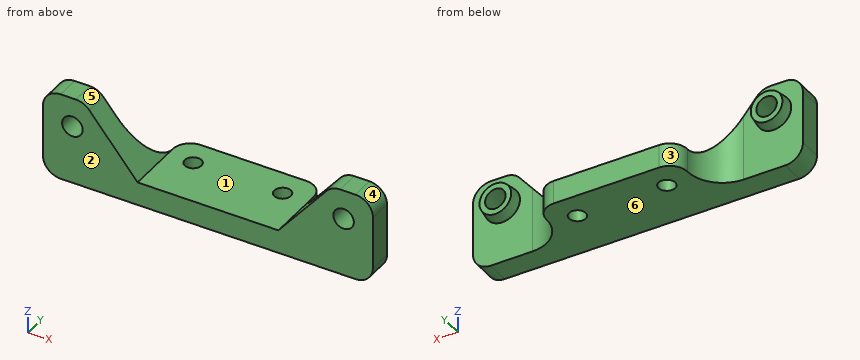
Autodesk Fusion 360 part; units mm, degrees
sketch "Sketch1" plane through (0, 0, 0) normal (0, 1, 0) x (1, 0, 0)
  line L0 (0, 0) -> (-28.109, 0)
  line L1 (-28.109, 0) -> (-28.109, -15)
  line L2 (-28.109, -15) -> (-21.109, -15)
  line L3 (-21.109, -15) -> (-12, -4)
  line L4 (-12, -4) -> (0, -4)
  line L5 (0, -4) -> (0, 0)
  circle A0 centre (-23.109, -10) radius 1.75
  line L6 (0, -1.75) -> (0, -22.5)
  line L7 (0, 0) -> (28.109, 0)
  line L8 (28.109, 0) -> (28.109, -15)
  line L9 (28.109, -15) -> (21.109, -15)
  line L10 (12, -4) -> (0, -4)
  line L11 (0, -4) -> (0, 0)
  line L12 (21.109, -15) -> (12, -4)
  circle A1 centre (23.109, -10) radius 1.75
  dimension "d1" = 23.109
  dimension "d2" = 3.5
  dimension "d3" = 10
  dimension "d4" = 5
  dimension "d5" = 5
  dimension "d6" = 7
  dimension "d8" = 12
  dimension "d9" = 4
extrude "Extrude1" add sketch "Sketch1" along normal blind 4
sketch "Sketch2" plane through (0, 4, 0) normal (0, 1, 0) x (-1, 0, 0)
  circle A0 centre (23.109, 10) radius 1.75
  circle A1 centre (-23.109, 10) radius 1.75
  line L0 (-28.109, 0) -> (28.109, 0)
  line L1 (28.109, 0) -> (28.109, 15)
  line L2 (28.109, 15) -> (21.109, 15)
  line L3 (21.109, 15) -> (12, 4)
  line L4 (12, 4) -> (-12, 4)
  line L5 (-12, 4) -> (-21.109, 15)
  line L6 (-21.109, 15) -> (-28.109, 15)
  line L7 (-28.109, 15) -> (-28.109, 0)
  line L8 (-12, 4) -> (12, 4)
  line L9 (12, 4) -> (12, 0)
  line L10 (12, 0) -> (-12, 0)
  line L11 (-12, 0) -> (-12, 4)
extrude "Extrude2" add sketch "Sketch2" along normal blind 9 contours L0 L4 L8 L9 L10 L11
sketch "Sketch3" plane through (0, 4, 0) normal (0, 1, 0) x (-1, 0, 0)
  line L0 (12, 4) -> (12, 0)
  line L1 (12, 0) -> (28.109, 0)
  line L2 (28.109, 0) -> (28.109, 15)
  line L3 (28.109, 15) -> (21.109, 15)
  line L4 (21.109, 15) -> (12, 4)
  circle A0 centre (23.109, 10) radius 1.75
  circle A1 centre (23.109, 10) radius 3
  line L5 (-12, 0) -> (-12, 4)
  line L6 (-12, 4) -> (-21.109, 15)
  line L7 (-21.109, 15) -> (-28.109, 15)
  line L8 (-28.109, 15) -> (-28.109, 0)
  line L9 (-28.109, 0) -> (-12, 0)
  circle A2 centre (-23.109, 10) radius 1.75
  circle A3 centre (-23.109, 10) radius 3
  dimension "d14" = 6
extrude "Extrude3" add sketch "Sketch3" along normal blind 2 contours A1 | A3
chamfer "Chamfer1" distance 0.3 distance2 2 2 edges at (25.906, 6, 8.9152) (-20.312, 6, 8.9152) measured on face at (20.5434, 6, 9.764) measured on face at (-25.6746, 6, 9.764)
sketch "Sketch4" plane through (0, 0, 4) normal (0, 0, 1) x (-1, 0, 0)
  line L0 (12, 0) -> (-12, 0)
  line L1 (-12, 0) -> (-12, -4)
  line L2 (-12, -4) -> (-12, -13)
  line L3 (-12, -13) -> (12, -13)
  line L4 (12, -13) -> (12, -4)
  line L5 (12, -4) -> (12, 0)
  line L6 (0, 0) -> (0, -19.3356) construction
  circle A0 centre (7.62, -8.5) radius 1.425
  circle A1 centre (-7.62, -8.5) radius 1.425
  dimension "d19" = 7.62
  dimension "d20" = 2.85
  dimension "d21" = 8.5
extrude "Extrude4" cut sketch "Sketch4" against normal blind 10 contours A0 | A1
fillet "Fillet1" radius 3 8 edges at (28.109, 2, 0) (28.109, 2, 15) (21.109, 2, 15) (-21.109, 2, 15) (-28.109, 2, 15) (-28.109, 2, 0) (12, 13, 2) (-12, 13, 2)
fillet "Fillet2" radius 6 2 edges at (12, 4, 2) (-12, 4, 2)
equation "d1 = ( 46.218 / 2 ) * 1 mm"
Work out the finished part from the listing and answer in its coordinate system (mm). Face numbers are marked on the shaded views. A direction names the side the tool comes from. Round coordinates to 2 decimals unless told otherwise and drop trailing zeros. Order: outer loops, then holes, each group sorted by start corner. A loop starts at its lowest first (then second) coordinate and runs counter-clockwise, first axis right, second up. Notation, with made-up numbers: M 59.5,41.5 L 91.5,41.5 A25 ccw 91.5,57.5 Z; hole C 47.25,86 d4. An arc over 180 degrees is marked long. Put each result on its own line as item: value. Start each with the question number.
Q1. Straight lines are drawn through the part: L1, parallel to X at y = 8.5, z = 2.5 (3 decimals); L2, parallel to Y at x = 7.62, z = 3.1 (3 decimals); L3, parallel to Z at x = -23, y = 1.5. For each, find the intervals that lie inside material, in ascending order. Write a range as [from, to].
Q2. A tool of negligible diameter and unlimited length cuts with its end or side. For the marked faces 5 and 6, from which of +Z, -Z, +X, -X, +Y, -Y can it reach the whole face along a straight path? Write none if from no direction.
Q3. Section B-B, the plane x = 7.62 is taken. Write down the section's boundary in (y, z) (3 decimals).
Q4. Flat-ended cylindrical pins translate along their axes: pin 1 (5 mm diameter, centred on x = -17.5, z = 8, fed in from +Y); pin 2 (3 mm diameter, centred on x = -16, y = 7, fed in from +Z). Find the tip coordinate at first contact, or state that the pin passes through.
Q5. Section D-D, the plane x = -3.5 is taken. Write down the section's boundary in (y, z).
Q6. For a pull along X with two mould halves and no side action, classify the marked faces 1, 2, 3 and 4 as pulls with the +X half, pulls with the -X half, needs draft (parallel to the pull), parting line crosses it, or undercut.
Q7. Section A-A, the plane y = 8.5 is taken. Write down the section's boundary in (x, z) (3 decimals).
Q8. Section C-C, the plane y = 5.25 is taken. Write down the section's boundary in (x, z).
Findings below:
1. L1: x = [-12.19, -9.045], [-6.195, 6.195], [9.045, 12.19]
1. L2: y = [0, 7.075], [9.925, 13]
1. L3: z = [0, 8.25], [11.75, 15]
2. face 5: +Z, +Y, -Y
2. face 6: -Z, +X, -X, +Y, -Y
3. outline: M 0,0 L 7.075,0 L 7.075,4 L 0,4 Z; M 9.925,0 L 13,0 L 13,4 L 9.925,4 Z
4. pin 1: stops at y = 4.79
4. pin 2: passes through
5. outline: M 0,0 L 13,0 L 13,4 L 0,4 Z
6. face 1: undercut
6. face 2: needs draft
6. face 3: pulls with the -X half
6. face 4: pulls with the +X half
7. outline: M -12.19,0 L -9.045,0 L -9.045,4 L -12,4 L -12.19,4.23 Z; M -6.195,0 L 6.195,0 L 6.195,4 L -6.195,4 Z; M 9.045,0 L 12.19,0 L 12.19,4.23 L 12,4 L 9.045,4 Z
8. outline: C -23.11,10 d5.63; M -14.33,0 L 14.33,0 L 14.33,6.82 L 12,4 L -12,4 L -14.33,6.82 Z; C 23.11,10 d5.63; hole C -23.11,10 d3.5; hole C 23.11,10 d3.5
